```python
from build123d import *

# Parameters (mm, degrees)
SKETCH_1_R      = 5
SKETCH_1_R_2    = 2.1
EXTRUDE_1_DEPTH = 3


with BuildPart() as part:
    # 草图1 → 凸台-拉伸1 (new body)
    with BuildSketch(Plane(origin=(0, 0, 40.05672841), x_dir=(-1, 0, 0), z_dir=(0, 0, -1))):
        with BuildLine():
            Line((83.25633153, -79.958506894), (11.650116444, 57.209335041))
            ThreePointArc((11.650116444, 57.209335041), (-11.219662978, 63.867129513), (-16.911730575, 40.738069772))
            Line((-16.911730575, 40.738069772), (65.946121215, -89.941091905))
            ThreePointArc((65.946121215, -89.941091905), (79.387248151, -93.248956728), (83.25633153, -79.958506894))
        make_face()
        with Locations((74.391553652, -84.586218334)):
            Circle(SKETCH_1_R, mode=Mode.SUBTRACT)
        with Locations((-14.924086576, 50.696801373)):
            Circle(SKETCH_1_R_2, mode=Mode.SUBTRACT)
        with Locations((-7.977715561, 60.481888482)):
            Circle(SKETCH_1_R_2, mode=Mode.SUBTRACT)
        with Locations((3.969603961, 59.358698272)):
            Circle(SKETCH_1_R_2, mode=Mode.SUBTRACT)
        with Locations((8.970552467, 48.450420955)):
            Circle(SKETCH_1_R_2, mode=Mode.SUBTRACT)
        with Locations((2.024181452, 38.665333847)):
            Circle(SKETCH_1_R_2, mode=Mode.SUBTRACT)
        with Locations((-9.92313807, 39.788524056)):
            Circle(SKETCH_1_R_2, mode=Mode.SUBTRACT)
    extrude(amount=EXTRUDE_1_DEPTH)


solid = part.part
```
Input: part model. Units: mm. Frame: model coordinates. Give positions to 0.01 mm unless a question says otherwise; leave off trailing zeros. Order: outer loops, then holes, each group sorted by start corner. A loop starts at its lowest first (then second) coordinate and runs counter-clockwise, first axis right, second up. Notation, with made-up numbers: (30.25, 68.5) - (82.25, 68.5) arc R19 ccw to (82.25, 74.5) - close; hole circle Ø11 at (34.25, 35). An arc over 180 degrees is marked (long way). Put each result on its own line as item: value.
Item 1: Section query A-A, the plane x = -73. Return loops of the section in (y, z), then the cut area to 3 significant figures.
Found:
outline: (-94.49, 37.06) - (-89.39, 37.06) - (-89.39, 40.06) - (-94.49, 40.06) - close; (-79.78, 37.06) - (-60.31, 37.06) - (-60.31, 40.06) - (-79.78, 40.06) - close
area: 73.7 mm^2
Item 2: Contact query for flat-ended pins moving along their axis: pin 1 (3.5 mm diameter, centred on x = 9.92, y = 39.79, fed in from +Z); pin 2 (1.5 mm diameter, centred on x = -64.5, z = 37.5, fed in from -Y). Output: stop coordinate, or through.
Found:
pin 1: passes through
pin 2: stops at y = -88.84
Item 3: Section query B-B, the plane z = 38. Return loops of the section in (x, y), then the cut area to 3 significant figures.
Found:
outline: (-83.26, -79.96) arc R10 ccw to (-65.95, -89.94) - (16.91, 40.74) arc R16.5 ccw (long way) to (-11.65, 57.21) - close; hole circle Ø10 at (-74.39, -84.59); hole circle Ø4.2 at (-8.97, 48.45); hole circle Ø4.2 at (-3.97, 59.36); hole circle Ø4.2 at (-2.02, 38.67); hole circle Ø4.2 at (7.98, 60.48); hole circle Ø4.2 at (9.92, 39.79); hole circle Ø4.2 at (14.92, 50.7)
area: 4,530 mm^2
Item 4: Section query C-C, the plane y = 35. Return loops of the section in (x, z), then the cut area to 3 significant figures.
Found:
outline: (-23.24, 37.06) - (13.27, 37.06) - (13.27, 40.06) - (-23.24, 40.06) - close
area: 110 mm^2
Item 5: Section query D-D, the plane x = -14. Return loops of the section in (y, z), then the cut area to 3 significant figures.
Found:
outline: (-8.01, 37.06) - (52.71, 37.06) - (52.71, 40.06) - (-8.01, 40.06) - close
area: 182 mm^2
Item 6: Draft query along Y for faces 1 (the cylindrical face through (10.89, 64.05, 38.58)), 2 (the cylindrical face through (10.38, 37.74, 38.58)), 3 (the flat face through (-32, -8, 37.057)). Return one class per face: +Y half, -Y half, draft (parallel to the pull), parting line (faces both ways), or undercut.
Found:
face 1: parting line
face 2: undercut
face 3: draft
Item 7: Ray query, L1, parallel to Y at x = -9, z = 38.25; L2, parallel to X at y = 57.5, z = 38.8; L3, parallel to Y at x = -55, z = 39.25. Return the intervals inside material, ascending. Write a range as from..to.
Found:
L1: y = -0.13..46.35, 50.55..60.92
L2: x = -11.49..-4.95, -2.99..17.45
L3: y = -72.68..-25.83
